```python
from build123d import *

# Parameters (mm, degrees)
F1_DEPTH      = 12.7
F3_D          = 15.875
F4_W          = 44.45
F4_H          = 31.75
F5_DEPTH      = 41.275
F8_START      = -19.05
F7_W          = 44.45
F7_H          = 15.875
F8_DEPTH      = 22.225
F6_W          = 25.4
F6_H          = 22.225
F9_DEPTH      = 31.751
F9_DEPTH_BACK = 38.101


with BuildPart() as f1:
    # F0 (on Top) → F1 (new body)
    with BuildSketch(Plane.XY):
        Polygon((120.65, 0), (0, 0), (0, -31.75), (38.1, -69.85), (82.55, -69.85), (120.65, -31.75), align=None)
    extrude(amount=F1_DEPTH)

    # F3 (through all)
    with Locations(Plane.XY.offset(12.7)):
        with Locations((19.05, -19.05), (101.6, -19.05)):
            Hole(F3_D / 2)

    # F4 (on face) → F5 (join)
    with BuildSketch(Plane.XY.offset(12.7)):
        with Locations((60.325, -15.875)):
            Rectangle(F4_W, F4_H)
    extrude(amount=F5_DEPTH)

    # F7 (on face) → F8 (join)
    with BuildSketch(Plane.XY.offset(53.975).offset(F8_START)):
        with Locations((60.325, -39.6875)):
            Rectangle(F7_W, F7_H)
    extrude(amount=-F8_DEPTH)

    # F6 (on face) → F9 (cut, two sides)
    with BuildSketch(Plane.XZ.offset(31.75)) as f9_sk:
        with Locations((69.85, 33.3375)):
            Rectangle(F6_W, F6_H)
    extrude(amount=-F9_DEPTH, mode=Mode.SUBTRACT)
    extrude(f9_sk.sketch, amount=F9_DEPTH_BACK, mode=Mode.SUBTRACT)


solid = f1.part
```
Verification items for the finished model (mm, model axes). A direction names the side the tool comes from. Give positions to 0.01 mm unless a question says otherwise; leave off trailing zeros. Loops run counter-clockwise (first coordinate to the right, second up) from the corner with the lowest first, then second, coordinate; pieces in that order, holes last. Notation, with made-up numbers: M 20,20 L 57,20 A13 cw 57,43 Z; hole C 50,81 d9. An arc over 180 degrees is marked long. One line per question, with ' | ' between items.
Item 1: Section check A-A, the plane x = 19.05. Record the cut outline in (y, z).
Completed:
outline: M -50.8,0 L -26.99,0 L -26.99,12.7 L -50.8,12.7 Z; M -11.11,0 L 0,0 L 0,12.7 L -11.11,12.7 Z
Item 2: Tool access check on faces 1 (the face through (57.15, -18, 33)), 2 (the face through (47, -40, 34.925)), 3 (the face through (82.55, -24, 18)), 4 (the face through (38.1, -19, 34)). Record the directions out of +Z, -Z, +X, -X, +Y, -Y that give a thin tool (end or side, any length) a straight path to the whole face; none if there is none.
Completed:
face 1: +X, +Y, -Y | face 2: +Z, +X, -X, -Y | face 3: +Z, +X, +Y, -Y | face 4: +Z, -X, +Y, -Y
Item 3: Section check B-B, the plane y = -7. Record the cut outline in (x, z) (3 decimals), plus the area to 3 significant figures.
Completed:
outline: M 0,0 L 120.65,0 L 120.65,12.7 L 82.55,12.7 L 82.55,22.225 L 57.15,22.225 L 57.15,44.45 L 82.55,44.45 L 82.55,53.975 L 38.1,53.975 L 38.1,12.7 L 0,12.7 Z | area: 2,800 mm^2
Item 4: Thickness scan on line 1 (X direction, y = -19, z = 4); line 2 (Z direction, x = 73.5, y = -14) (3 decimals); line 3 (Z direction, x = 32.5, y = -26). Record the ranges inside material, lowest first. Write a range as [from, to].
Completed:
line 1: x = [0, 11.11], [26.99, 93.66], [109.54, 120.65] | line 2: z = [0, 22.225], [44.45, 53.975] | line 3: z = [0, 12.7]
Item 5: Draft check along Z on faces 5 (the face through (101.3, -51.1, 6.3)), 6 (the face through (60, -16, 53.975)), 7 (the face through (70, -23, 22.225)), 8 (the face through (70, -16, 44.45)). Enter one of: +Z half, -Z half, draft (parallel to the pull), parting line (faces both ways), or undercut.
Completed:
face 5: draft | face 6: +Z half | face 7: undercut | face 8: undercut
Item 6: Section check C-C, the plane z = 7. State how many separate pieces and enclosed holes the cut face has, plus the area to 3 significant figures.
Completed:
separate pieces: 1 | enclosed holes: 2 | area: 6,580 mm^2
Item 7: Depth check by flat-ended pin: P1, Ø6, axis at x = 40, y = -15, coming from the -Z side; P2, Ø18, axis at x = 58, z = 25, coming from the -Y side (3 decimals); P3, Ø3, axis at y = -25.5, z = 16, coming from the +X side; P4, Ø5.5, axis at x = 66, z = 45, coming from the -Y side. Enter the tip coordinate at first touch or a pass-through.
Completed:
P1: stops at z = 0 | P2: stops at y = -47.625 | P3: stops at x = 82.55 | P4: stops at y = -31.75
